from build123d import *

# Parameters (mm, degrees)
F1_DEPTH = 63.5
F2_DEPTH = 25.4
F3_DEPTH = 7.9375


with BuildPart() as f1:
    # F0 (on Front) → F1 (new body, symmetric)
    with BuildSketch(Plane.XZ):
        Polygon((-41.275, -9.525), (41.275, -9.525), (41.275, 9.525), (41.0909965214, 9.525), (22.225, 9.525), (-41.275, 9.525), align=None)
    extrude(amount=F1_DEPTH, both=True)

    # F0 (on Front) → F2 (join, symmetric)
    with BuildSketch(Plane.XZ):
        with BuildLine():
            Line((22.225, 9.525), (41.0909965214, 9.525))
            Line((41.0909965214, 9.525), (41.0909965214, 27.0002))
            ThreePointArc((41.0909965214, 27.0002), (45.7945697412, 38.3556302588), (57.15, 43.0592034786))
            Line((57.15, 43.0592034786), (60.325, 43.0592034786))
            Line((60.325, 43.0592034786), (60.325, 61.9252))
            Line((60.325, 61.9252), (57.15, 61.9252))
            ThreePointArc((57.15, 61.9252), (32.4542956671, 51.6959043329), (22.225, 27.0002))
            Line((22.225, 27.0002), (22.225, 9.525))
        make_face()
        Polygon((85.725, 61.9252), (60.325, 61.9252), (60.325, 43.0592034786), (60.325, 42.8752), (85.725, 42.8752), align=None)
    extrude(amount=F2_DEPTH, both=True)

    # F0 (on Front) → F3 (join, symmetric)
    with BuildSketch(Plane.XZ):
        with BuildLine():
            add(Edge.make_bspline(
                [(-41.275, 9.525), (-30.462404713, 45.4226024449), (15.5969550833, 63.5012462735), (57.15, 61.9252)],
                knots=[0, 0, 0, 0, 111.5045361635, 111.5045361635, 111.5045361635, 111.5045361635], degree=3))
            Line((-41.275, 9.525), (22.225, 9.525))
            Line((22.225, 9.525), (22.225, 27.0002))
            ThreePointArc((22.225, 27.0002), (32.4542956671, 51.6959043329), (57.15, 61.9252))
        make_face()
    extrude(amount=F3_DEPTH, both=True)

    # F0 (on Front) → F4 (revolve)
    with BuildSketch(Plane.XZ):
        Polygon((85.725, 66.675), (85.725, 61.9252), (85.725, 42.8752), (85.725, 38.1), (111.125, 38.1), (111.125, 66.675), align=None)
    revolve(axis=Axis((85.725, 0, 52.3875), (0, 0, 1)))


solid = f1.part
Input: part model. Units: mm. Frame: model coordinates. A direction names the side the tool comes from. Give positions to 0.01 mm unless a question says otherwise; leave off trailing zeros. Order: outer loops, then holes, each group sorted by start corner. A loop starts at its lowest first (then second) coordinate and runs counter-clockwise, first axis right, second up.
Q1. Section B-B on y = -49.5. Output: boundary loops of the cut face in (x, z) (3 decimals), and give its area (3 significant figures).
Checked values:
outline: (-41.275, -9.525) - (41.275, -9.525) - (41.275, 9.525) - (-41.275, 9.525) - close
area: 1,570 mm2
Q2. Section A-A on x = 71. Output: boundary loops of the cut face in (y, z) (3 decimals).
Checked values:
outline: (-25.4, 42.875) - (-20.696, 42.875) - (-20.696, 38.1) - (20.696, 38.1) - (20.696, 42.875) - (25.4, 42.875) - (25.4, 61.925) - (20.696, 61.925) - (20.696, 66.675) - (-20.696, 66.675) - (-20.696, 61.925) - (-25.4, 61.925) - close
Q3. Ray query, probe 1 along Z at (x, y) = (13, -50) (3 decimals); probe 2 along X at (y, z) = (-14.5, 26.5) (3 decimals); probe 3 along Y at (x, z) = (24.5, 32). Return the intervals inside material, ascending.
Checked values:
probe 1: z = -9.525 to 9.525
probe 2: x = 22.225 to 41.091
probe 3: y = -25.4 to 25.4
Q4. Set-up query: faces 1 (the flat face through (22.225, 17, 18)), 2 (the flat face through (46, -25.4, 42)), 3 (the flat face through (65, 19, 42.875)). Return all of +Z, -Z, +X, -X, +Y, -Y with unobstructed straight access to the full face (end or side cutting, diameter ignored); none if empty.
Checked values:
face 1: +Z, -X, +Y
face 2: +Z, +X, -X, -Y
face 3: -Z, +Y
Q5. Draft query along X for faces 4 (the flat face through (-1, 63.5, 0)), 5 (the flat face through (41.091, 0, 18)), 6 (the cylindrical face through (32.73, -16.79, 51.97)), 7 (the cylindrical face through (45.67, -0.36, 38.23)). Return one class per face: +X half, -X half, draft (parallel to the pull), parting line (faces both ways), or undercut.
Checked values:
face 4: draft
face 5: +X half
face 6: -X half
face 7: undercut
Q6. Section C-C on x = 91.5. Output: boundary loops of the cut face in (y, z) (3 decimals), and give its area (3 significant figures).
Checked values:
outline: (-24.735, 38.1) - (24.735, 38.1) - (24.735, 66.675) - (-24.735, 66.675) - close
area: 1,410 mm2
Q7. Contact query for flat-ended pins moving along their axis: pin 1 Ø10 at (y, z) = (-8, 38) entering from +X; pin 2 Ø15 at (y, z) = (-3.5, 0.5) entering from +X (3 decimals); pin 3 Ø12.5 at (x, y) = (69.5, -11.5) entering from -Z. Output: stop coordinate, or through.
Checked values:
pin 1: stops at x = 110.95
pin 2: stops at x = 41.275
pin 3: stops at z = 38.1
